```python
from build123d import *

# Parameters (mm, degrees)
F0_R     = 3.05
F0_R_2   = 2.05
F1_DEPTH = 5
F2_DEPTH = 2
F3_DEPTH = 0.5


with BuildPart() as f1:
    # F0 (on Top) → F1 (new body)
    with BuildSketch(Plane.XY):
        with Locations((-31.2889043277, -23.0932135019)):
            Circle(F0_R)
        with Locations((-31.2889043277, -23.0932135019)):
            Circle(F0_R_2, mode=Mode.SUBTRACT)
    extrude(amount=F1_DEPTH)

    # F0 (on Top) → F2 (join)
    with BuildSketch(Plane.XY):
        with BuildLine():
            ThreePointArc((-27.2466277414, -23.3432135019), (-27.2408356416, -23.2182731388), (-27.2389043277, -23.0932135019))
            ThreePointArc((-27.2389043277, -23.0932135019), (-27.2408356416, -22.9681538651), (-27.2466277414, -22.8432135019))
            ThreePointArc((-27.2466277414, -22.8432135019), (-35.3389043277, -23.0932135019), (-27.2466277414, -23.3432135019))
        make_face()
        with Locations((-31.2889043277, -23.0932135019)):
            Circle(F0_R, mode=Mode.SUBTRACT)
        with Locations((-31.2889043277, -23.0932135019)):
            Circle(F0_R_2)
    extrude(amount=F2_DEPTH)



with BuildPart() as f1b:
    # F0 (on Top) → F1, piece 2 (new body)
    with BuildSketch(Plane.XY):
        with Locations((-22.6889043277, -23.0932135019)):
            Circle(F0_R)
        with Locations((-22.6889043277, -23.0932135019)):
            Circle(F0_R_2, mode=Mode.SUBTRACT)
    extrude(amount=F1_DEPTH)

    # F0 (on Top) → F2, piece 2 (join)
    with BuildSketch(Plane.XY):
        with BuildLine():
            ThreePointArc((-18.6466277414, -22.8432135019), (-22.6889043277, -19.0432135019), (-26.731180914, -22.8432135019))
            ThreePointArc((-26.731180914, -22.8432135019), (-26.7389043277, -23.0932135019), (-26.731180914, -23.3432135019))
            ThreePointArc((-26.731180914, -23.3432135019), (-22.6889043277, -27.1432135019), (-18.6466277414, -23.3432135019))
            ThreePointArc((-18.6466277414, -23.3432135019), (-18.6408356416, -23.2182731388), (-18.6389043277, -23.0932135019))
            ThreePointArc((-18.6389043277, -23.0932135019), (-18.6408356416, -22.9681538651), (-18.6466277414, -22.8432135019))
        make_face()
        with Locations((-22.6889043277, -23.0932135019)):
            Circle(F0_R, mode=Mode.SUBTRACT)
        with Locations((-22.6889043277, -23.0932135019)):
            Circle(F0_R_2)
    extrude(amount=F2_DEPTH)


with BuildPart() as f1c:
    # F0 (on Top) → F1, piece 3 (new body)
    with BuildSketch(Plane.XY):
        with Locations((-14.0889043277, -23.0932135019)):
            Circle(F0_R)
        with Locations((-14.0889043277, -23.0932135019)):
            Circle(F0_R_2, mode=Mode.SUBTRACT)
    extrude(amount=F1_DEPTH)

    # F0 (on Top) → F2, piece 3 (join)
    with BuildSketch(Plane.XY):
        with BuildLine():
            ThreePointArc((-10.0466277414, -22.8432135019), (-14.0889043277, -19.0432135019), (-18.131180914, -22.8432135019))
            ThreePointArc((-18.131180914, -22.8432135019), (-18.1389043277, -23.0932135019), (-18.131180914, -23.3432135019))
            ThreePointArc((-18.131180914, -23.3432135019), (-14.0889043277, -27.1432135019), (-10.0466277414, -23.3432135019))
            ThreePointArc((-10.0466277414, -23.3432135019), (-10.0408356416, -23.2182731388), (-10.0389043277, -23.0932135019))
            ThreePointArc((-10.0389043277, -23.0932135019), (-10.0408356416, -22.9681538651), (-10.0466277414, -22.8432135019))
        make_face()
        with Locations((-14.0889043277, -23.0932135019)):
            Circle(F0_R, mode=Mode.SUBTRACT)
        with Locations((-14.0889043277, -23.0932135019)):
            Circle(F0_R_2)
    extrude(amount=F2_DEPTH)


with BuildPart() as f1d:
    # F0 (on Top) → F1, piece 4 (new body)
    with BuildSketch(Plane.XY):
        with Locations((-5.4889043277, -23.0932135019)):
            Circle(F0_R)
        with Locations((-5.4889043277, -23.0932135019)):
            Circle(F0_R_2, mode=Mode.SUBTRACT)
    extrude(amount=F1_DEPTH)

    # F0 (on Top) → F2, piece 4 (join)
    with BuildSketch(Plane.XY):
        with BuildLine():
            ThreePointArc((-1.4389043277, -23.0932135019), (-5.3638446908, -19.0451448159), (-9.531180914, -22.8432135019))
            ThreePointArc((-9.531180914, -22.8432135019), (-9.5389043277, -23.0932135019), (-9.531180914, -23.3432135019))
            ThreePointArc((-9.531180914, -23.3432135019), (-5.3638446908, -27.141282188), (-1.4389043277, -23.0932135019))
        make_face()
        with Locations((-5.4889043277, -23.0932135019)):
            Circle(F0_R, mode=Mode.SUBTRACT)
        with Locations((-5.4889043277, -23.0932135019)):
            Circle(F0_R_2)
    extrude(amount=F2_DEPTH)


with BuildPart() as f1_1:
    add(f1.part)

    add(f1b.part)  # F3 merges F1b

    add(f1c.part)  # F3 merges F1c

    add(f1d.part)  # F3 merges F1d
    # F0 (on Top) → F3 (join)
    with BuildSketch(Plane.XY):
        with BuildLine():
            ThreePointArc((-27.2466277414, -22.8432135019), (-27.2408356416, -22.9681538651), (-27.2389043277, -23.0932135019))
            ThreePointArc((-27.2389043277, -23.0932135019), (-27.2408356416, -23.2182731388), (-27.2466277414, -23.3432135019))
            Line((-27.2466277414, -23.3432135019), (-26.731180914, -23.3432135019))
            ThreePointArc((-26.731180914, -23.3432135019), (-26.7389043277, -23.0932135019), (-26.731180914, -22.8432135019))
            Line((-26.731180914, -22.8432135019), (-27.2466277414, -22.8432135019))
        make_face()
        with BuildLine():
            Line((-18.131180914, -22.8432135019), (-18.6466277414, -22.8432135019))
            ThreePointArc((-18.6466277414, -22.8432135019), (-18.6408356416, -22.9681538651), (-18.6389043277, -23.0932135019))
            ThreePointArc((-18.6389043277, -23.0932135019), (-18.6408356416, -23.2182731388), (-18.6466277414, -23.3432135019))
            Line((-18.6466277414, -23.3432135019), (-18.131180914, -23.3432135019))
            ThreePointArc((-18.131180914, -23.3432135019), (-18.1389043277, -23.0932135019), (-18.131180914, -22.8432135019))
        make_face()
        with BuildLine():
            Line((-9.531180914, -22.8432135019), (-10.0466277414, -22.8432135019))
            ThreePointArc((-10.0466277414, -22.8432135019), (-10.0408356416, -22.9681538651), (-10.0389043277, -23.0932135019))
            ThreePointArc((-10.0389043277, -23.0932135019), (-10.0408356416, -23.2182731388), (-10.0466277414, -23.3432135019))
            Line((-10.0466277414, -23.3432135019), (-9.531180914, -23.3432135019))
            ThreePointArc((-9.531180914, -23.3432135019), (-9.5389043277, -23.0932135019), (-9.531180914, -22.8432135019))
        make_face()
    extrude(amount=F3_DEPTH)


solid = f1_1.part
```
Geometry: final body of the model. Coordinates: model frame, mm. A direction names the side the tool comes from. Coordinates: 2 decimals unless noted, no trailing zeros. Loops run counter-clockwise (first coordinate to the right, second up) from the corner with the lowest first, then second, coordinate; pieces in that order, holes last. Notation, with made-up numbers: (60, 11) -> (86, 11) arc R32 cw to (86, 50) -> close; hole circle Ø4 at (-5.5, 64.5). An arc over 180 degrees is marked (long way). Use a Markdown table: item, result. Add a question column.
(1) Section query D-D, the plane x = -14.5. Return loops of the section in (y, z).
(2) Line query: line 1 along X through (y, z) = (-23.5, 1.15); line 2 along X through (y, z) = (-20.5, 4.05); line 3 along Z through (x, y) = (-23.5, -22). Output: solid intervals per line, ascending.
(3) Pin query (flat end, axial travel): pin 1 Ø3 at (x, z) = (-20.5, 0.5) entering from +Y; pin 2 Ø3 at (x, y) = (-22.5, -23) entering from -Z; pin 3 Ø1 at (y, z) = (-20.5, 3) entering from -X; pin 4 Ø2 at (x, y) = (-22, -22.5) entering from +Z. Return the tip coordinate at first contact, or that it passes through.
(4) Section query C-C, the plane y = -19.5. Return loops of the section in (x, z), plus the area to 3 significant figures.
(5) Access query for faces 3 (the cylindrical face through (-14.5, -25.1, 3.5)), 4 (the flat face through (-3, -24, 5)). Directions: +Z, -Z, +X, -X, +Y, -Y. A direction counts if a zero-diameter tool reaches every point of the face in a straight line with its end or side. Return the directions, or none.
(6) Section query B-B, the plane z = 1.5. Return loops of the section in (x, y), plus the area to 3 significant figures.
(7) Mould query, pull axis X, two halves, no side actions, for faces 1 (the flat face through (-23, -23, 2)), 2 (the flat face through (-12, -24, 5)). Classes: pulls with the +X half, pulls with the -X half, needs draft (parallel to the pull), parting line crosses it, or undercut.
(8) Section query A-A, the plane z = 3. Return loops of the section in (x, y).
Answer:
| question | item | result |
|---|---|---|
| 1 | outline | (-27.12, 0) -> (-19.06, 0) -> (-19.06, 2) -> (-20.07, 2) -> (-20.07, 5) -> (-21.08, 5) -> (-21.08, 2) -> (-25.1, 2) -> (-25.1, 5) -> (-26.12, 5) -> (-26.12, 2) -> (-27.12, 2) -> close |
| 2 | line 1 | x = -35.32 to -27.26, -26.72 to -18.66, -18.12 to -10.06, -9.52 to -1.46 |
| 2 | line 2 | x = -32.89 to -29.68, -24.29 to -21.08, -15.69 to -12.48, -7.09 to -3.88 |
| 2 | line 3 | z = 0 to 2 |
| 3 | pin 1 | stops at y = -19.1 |
| 3 | pin 2 | stops at z = 0 |
| 3 | pin 3 | stops at x = -33.51 |
| 3 | pin 4 | stops at z = 2 |
| 4 | outline | (-33.16, 0) -> (-29.42, 0) -> (-29.42, 2) -> (-33.16, 2) -> close; (-24.56, 0) -> (-20.82, 0) -> (-20.82, 2) -> (-24.56, 2) -> close; (-15.96, 0) -> (-12.22, 0) -> (-12.22, 2) -> (-15.96, 2) -> close; (-7.36, 0) -> (-3.62, 0) -> (-3.62, 2) -> (-7.36, 2) -> close |
| 4 | area | 29.9 mm^2 |
| 5 | face 3 | +Z |
| 5 | face 4 | +Z, +X, -X, +Y, -Y |
| 6 | outline | circle Ø8.1 at (-31.29, -23.09); circle Ø8.1 at (-22.69, -23.09); circle Ø8.1 at (-14.09, -23.09); circle Ø8.1 at (-5.49, -23.09) |
| 6 | area | 206 mm^2 |
| 7 | face 1 | undercut |
| 7 | face 2 | needs draft |
| 8 | outline | circle Ø6.1 at (-31.29, -23.09); circle Ø6.1 at (-22.69, -23.09); circle Ø6.1 at (-14.09, -23.09); circle Ø6.1 at (-5.49, -23.09); hole circle Ø4.1 at (-31.29, -23.09); hole circle Ø4.1 at (-22.69, -23.09); hole circle Ø4.1 at (-14.09, -23.09); hole circle Ø4.1 at (-5.49, -23.09) |
